Model file for the job. Use its own axes, mm. Coordinates: 2 decimals unless noted, no trailing zeros. Write each loop counter-clockwise with the first axis right and the second up, starting at its lowest first coordinate (ties: lowest second). Pieces come first, ordered by that corner, then holes. Notation, with made-up numbers: (59, -26) - (91, -26) arc R18 cw to (91, -10) - close; hole circle Ø11 at (17.25, 61.5). An arc over 180 degrees is marked (long way). Put each result on its own line as item: value. Start each with the question number.
1. Saw through at A-A, the plane x = 0. Write the cut outline in (y, z).
2. Saw through at C-C, the plane y = -17.5. Write the cut outline in (x, z).
3. Saw through at B-B, the plane y = -33.5. Write the cut outline in (x, z), plus the area to 3 significant figures.
4. Drop flat-ended pins along their axis: P1, Ø8, axis at y = -33, z = 43, coming from the +X side; P2, Ø10, axis at x = 36.5, y = -25, coming from the -Z side; P3, Ø5, axis at x = 54.5, y = -31, coming from the +Z side. Give the stop position or say it passes through.
5. Drill centre lines: L1, parallel to Y at x = -57, z = -20.5; L2, parallel to Y at x = -49.5, z = 22.5; L3, parallel to Z at x = -20.5, y = -31. Where is each one in solid material? Low to high. Write a range as from..to.
```python
from build123d import *

# Parameters (mm, degrees)
F0_R       = 73.8450197524
F1_DEPTH   = 50.8
F2_R       = 73.8450197524
F2_R_2     = 53.9474257016
F3_DEPTH   = 50.546
F1_FACE1_R = 73.8450197524
F1_FACE_R  = 53.9474257016


with BuildPart() as f1:
    # F0 (on Front) → F1 (new body)
    with BuildSketch(Plane.XZ):
        Circle(F0_R)
    extrude(amount=F1_DEPTH)

    # F2 (on face) → F3 (cut)
    with BuildSketch(Plane.XZ.offset(50.8)):
        Circle(F2_R)
        Circle(F2_R_2, mode=Mode.SUBTRACT)
    extrude(amount=-F3_DEPTH, mode=Mode.SUBTRACT)

    # F1_face1 (on face) → F4 section 0
    with BuildSketch(Plane(origin=(0, 0, 0), x_dir=(1, 0, 0), z_dir=(0, 1, 0))):
        Circle(F1_FACE1_R)
    # F1_face (on face) → F4 section 1
    with BuildSketch(Plane.XZ.offset(50.8)):
        Circle(F1_FACE_R)
    loft()


solid = f1.part
```
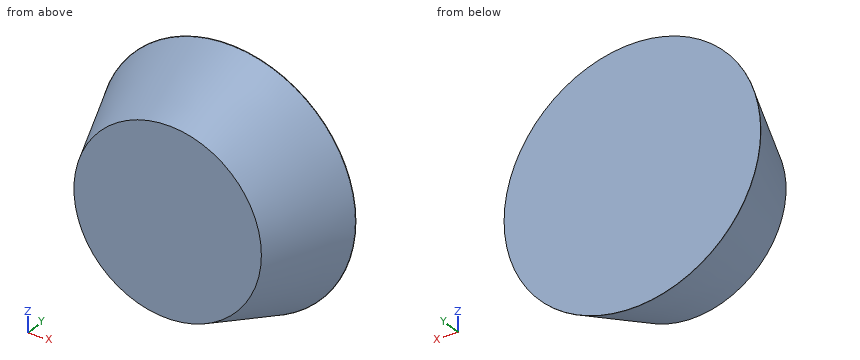
Final values:
1. outline: (-50.8, -53.95) - (-0.25, -73.75) - (-0.25, -73.85) - (0, -73.85) - (0, 73.85) - (-0.25, 73.85) - (-0.25, 73.75) - (-50.8, 53.95) - close
2. outline: circle Ø133.98 at (0, 0)
3. outline: circle Ø121.45 at (0, 0)
3. area: 11,600 mm²
4. P1: stops at x = 47.37
4. P2: stops at z = -56.56
4. P3: stops at z = 33.62
5. L1: y = -33.88..0
5. L2: y = -49.71..0
5. L3: z = -58.2..58.2
